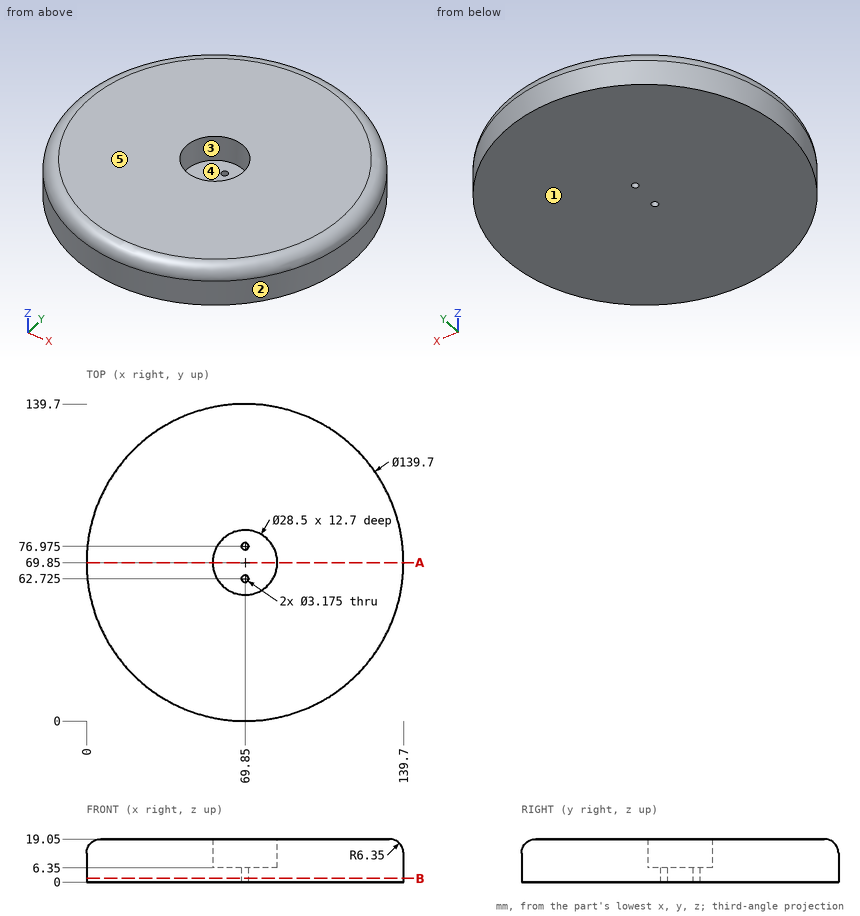
Answer from the drawing. Dimensions are ordinates in mm from the lowest x, y and z of the part. A direction names the side the tool comes from. Round coordinates to 2 decimals unless told otherwise and drop trailing zeros. Write each loop counter-clockwise with the first axis right and the second up, starting at its lowest first coordinate (ties: lowest second). Pieces come first, ordered by that corner, then holes. Notation, with made-up numbers: M -13,19 L 34,19 A11 cw 34,37 Z; hole C 39,-11 d1. An arc over 180 degrees is marked long. Write each question's results on one line, items separated by ' | '. Start each with the question number.
Item 1: Flat-ended cylindrical pins translate along their axes: pin 1 Ø5 at (x, y) = (69.85, 62.72) entering from +Z; pin 2 Ø12 at (x, y) = (117.5, 16.5) entering from +Z; pin 3 Ø6 at (x, z) = (82.5, 12.5) entering from -Y. Find the tip coordinate at first contact, or state that the pin passes through.
Item 2: A cutting plane is placed at B-B on z = 1.75. State how many separate pieces and enclosed holes the cut face has, and give its area (3 significant figures).
Item 3: For a pull along X with two mould halves and no side action, classify the marked faces 1, 2 and 3 as pulls with the +X half, pulls with the -X half, needs draft (parallel to the pull), parting line crosses it, or undercut.
Item 4: A cutting plane is placed at A-A on y = 69.85. Write down the section's boundary in (x, z), and give its area (3 significant figures).
Item 5: Straight lines are drawn through the part: L1, parallel to Y at x = 69.85, z = 2; L2, parallel to Y at x = 70, z = 8.25. For each, find the intervals that lie inside material, in ascending order. Write a range as [from, to].
Item 6: For the marked faces 4 and 5, determine the directions among +Z, -Z, +X, -X, +Y, -Y from which every point of the face is accessible in a straight line to the end or side of a thin tool.
Check sheet entries:
1) pin 1: z = 6.35 | pin 2: z = 18.72 | pin 3: y = 0.67
2) separate pieces: 1 | enclosed holes: 2 | area: 15,300 mm²
3) face 1: needs draft | face 2: parting line crosses it | face 3: undercut
4) outline: M 0,0 L 139.7,0 L 139.7,12.7 A6.35 ccw 133.35,19.05 L 84.1,19.05 L 84.1,6.35 L 55.6,6.35 L 55.6,19.05 L 6.35,19.05 A6.35 ccw 0,12.7 Z | area: 2,280 mm²
5) L1: [0, 61.14], [64.31, 75.39], [78.56, 139.7] | L2: [0, 55.6], [84.1, 139.7]
6) face 4: +Z | face 5: +Z, +X, -X, +Y, -Y
